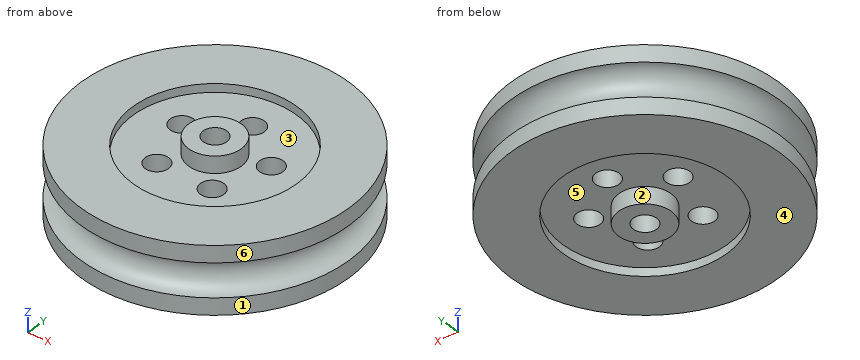
from build123d import *

# Parameters (mm, degrees)
SKETCH2_R           = 16
SKETCH2_R_2         = 1.4
BOSS_EXTRUDE1_DEPTH = 4
SKETCH3_R           = 9.8
CUT_EXTRUDE1_DEPTH  = 1
SKETCH6_R           = 3.15
SKETCH6_R_2         = 1.4
BOSS_EXTRUDE2_DEPTH = 2
SKETCH4_R           = 1.4
CUT_EXTRUDE2_DEPTH  = 25
CIRPATTERN1_COUNT   = 5
SKETCH5_R           = 2


with BuildPart() as part:
    # Sketch2 → Boss-Extrude1 (new, symmetric)
    with BuildSketch(Plane.XY):
        Circle(SKETCH2_R)
        Circle(SKETCH2_R_2, mode=Mode.SUBTRACT)
    extrude(amount=BOSS_EXTRUDE1_DEPTH, both=True)

    # Sketch3 → Cut-Extrude1 (cut)
    with BuildSketch(Plane.XY.offset(4)):
        Circle(SKETCH3_R)
    cut_extrude1 = extrude(amount=-CUT_EXTRUDE1_DEPTH, mode=Mode.SUBTRACT)

    # Sketch6 → Boss-Extrude2 (add)
    with BuildSketch(Plane.XY.offset(3)):
        Circle(SKETCH6_R)
        Circle(SKETCH6_R_2, mode=Mode.SUBTRACT)
    boss_extrude2 = extrude(amount=BOSS_EXTRUDE2_DEPTH)

    # Mirror1: Cut-Extrude1, Boss-Extrude2 across plane
    add(cut_extrude1.mirror(Plane.XY), mode=Mode.SUBTRACT)
    add(boss_extrude2.mirror(Plane.XY))

    # Sketch4 → Cut-Extrude2 (cut, through all)
    with BuildSketch(Plane.XY.offset(3)):
        with Locations((0, 5.6)):
            Circle(SKETCH4_R)
    cut_extrude2 = extrude(amount=-CUT_EXTRUDE2_DEPTH, mode=Mode.SUBTRACT)

    # CirPattern1: Cut-Extrude2 ×5 about axis
    cirpattern1_axis = Axis((0, 0, 0), (0, 0, 1))
    for i in range(1, CIRPATTERN1_COUNT):
        add(cut_extrude2.rotate(cirpattern1_axis, i * 360 / CIRPATTERN1_COUNT), mode=Mode.SUBTRACT)

    # Sketch5 → Cut-Revolve1 (revolve, cut)
    with BuildSketch(Plane(origin=(0, 0, 0), x_dir=(1, 0, 0), z_dir=(0, 1, 0)), mode=Mode.PRIVATE) as cut_revolve1_sk:
        with Locations((16, 0)):
            Circle(SKETCH5_R)
    revolve(cut_revolve1_sk.sketch.rotate(Axis((0, 0, -19.267509915), (0, 0, 1)), 180), axis=Axis((0, 0, -19.267509915), (0, 0, 1)), mode=Mode.SUBTRACT)


solid = part.part
Work out the finished part from the listing and answer in its coordinate system (mm). Face numbers are marked on the shaded views. A direction names the side the tool comes from. Give positions to 0.01 mm unless a question says otherwise; leave off trailing zeros. Loops run counter-clockwise (first coordinate to the right, second up) from the corner with the lowest first, then second, coordinate; pieces in that order, holes last. Notation, with made-up numbers: (-29, 86) -> (-23, 86) arc R27 ccw to (-23, 125) -> close; hole circle Ø11 at (23.5, 38). An arc over 180 degrees is marked (long way). Use a Markdown table: item, result. Add a question column.
1) The part is cut by section B-B, the plane z = 0.75. Determine the outline of the cut face in (x, y).
2) Consider line 1 along Y through (x, z) = (0, -3.95); line 2 along X through (y, z) = (-1, 3.75); line 3 along Y through (x, z) = (0, -4.2). Determine where each line is inside the solid, lowest interval first.
3) Each of these flat-tipped pins is pushed along its axis until it touches: P1, Ø1.7, axis at x = -5.33, y = 1.73, coming from the +Z side; P2, Ø6, axis at y = 12, z = -0.5, coming from the -X side; P3, Ø3, axis at x = 5.33, y = 1.73, coming from the +Z side; P4, Ø4, axis at y = 8, z = -2, coming from the -X side. Where does it stop, or does it pass through?
4) Which of the six approach directions +Z, -Z, +X, -X, +Y, -Y give full straight-line access (tool end or side, diameter ignored) to the marked faces 1, 2 and 3?
5) The part is cut by section A-A, the plane x = 0. Count the separate pieces of the cut face and the enclosed holes in it, plus the area to 3 significant figures.
6) For a pull along X with two mould halves and no side action, classify the marked faces 4, 5 and 6 as +X half, -X half, draft (parallel to the pull), parting line (faces both ways), or undercut.
7) The part is cut by section C-C, the plane z = 2.5. Determine the outline of the cut face in (x, y), plus the area to 3 significant figures.
Reported:
| question | item | result |
|---|---|---|
| 1 | outline | circle Ø28.29 at (0, 0); hole circle Ø2.8 at (-5.33, 1.73); hole circle Ø2.8 at (-3.29, -4.53); hole circle Ø2.8 at (0, 0); hole circle Ø2.8 at (0, 5.6); hole circle Ø2.8 at (3.29, -4.53); hole circle Ø2.8 at (5.33, 1.73) |
| 2 | line 1 | y = -16 to -9.8, -3.15 to -1.4, 1.4 to 3.15, 9.8 to 16 |
| 2 | line 2 | x = -15.97 to -9.75, -2.99 to -0.98, 0.98 to 2.99, 9.75 to 15.97 |
| 2 | line 3 | y = -3.15 to -1.4, 1.4 to 3.15 |
| 3 | P1 | passes through |
| 3 | P2 | stops at x = -12.95 |
| 3 | P3 | stops at z = 3 |
| 3 | P4 | stops at x = -14.83 |
| 4 | face 1 | +Z, -Z |
| 4 | face 2 | -Z |
| 4 | face 3 | +Z |
| 5 | separate pieces | 3 |
| 5 | enclosed holes | 0 |
| 5 | area | 185 mm^2 |
| 6 | face 4 | draft |
| 6 | face 5 | undercut |
| 6 | face 6 | parting line |
| 7 | outline | circle Ø32 at (0, 0); hole circle Ø2.8 at (-5.33, 1.73); hole circle Ø2.8 at (-3.29, -4.53); hole circle Ø2.8 at (0, 0); hole circle Ø2.8 at (0, 5.6); hole circle Ø2.8 at (3.29, -4.53); hole circle Ø2.8 at (5.33, 1.73) |
| 7 | area | 767 mm^2 |
